from build123d import *

# Parameters (mm, degrees)
SKETCH1_R                = 95.25
BOSS_EXTRUDE1_DEPTH      = 482.6
SKETCH4_R                = 95.25
F_7_PERCENT_ULLAGE_DEPTH = 62.484


with BuildPart() as part:
    # Sketch1 → Boss-Extrude1 (new body)
    with BuildSketch(Plane(origin=(0, 0, 0), x_dir=(1, 0, 0), z_dir=(0, 1, 0))):
        Circle(SKETCH1_R)
    extrude(amount=BOSS_EXTRUDE1_DEPTH)

    # Sketch2 → Revolve1 (revolve)
    with BuildSketch(Plane(origin=(0, 0, 0), x_dir=(0, 0, -1), z_dir=(1, 0, 0))):
        with BuildLine():
            Line((0, 544.576), (0, 482.6))
            Line((0, 482.6), (95.25, 482.6))
            add(Edge.make_bspline(
                [(95.25, 482.6), (95.25, 544.576), (0, 544.576)],
                knots=[0, 0, 0, 1.570796327, 1.570796327, 1.570796327], degree=2, weights=[1, 0.707106781, 1]))
        make_face()
    revolve(axis=Axis((0, 544.576, 0), (0, -1, 0)))

    # Sketch3 → Revolve2 (revolve)
    with BuildSketch(Plane(origin=(0, 0, 0), x_dir=(0, 0, -1), z_dir=(1, 0, 0))):
        with BuildLine():
            Line((0, -59.69), (0, 0))
            Line((0, 0), (95.25, 0))
            add(Edge.make_bspline(
                [(0, -59.69), (95.25, -59.69), (95.25, 0)],
                knots=[4.71238898, 4.71238898, 4.71238898, 6.283185307, 6.283185307, 6.283185307], degree=2, weights=[1, 0.707106781, 1]))
        make_face()
    revolve(axis=Axis((0, -59.69, 0), (0, 1, 0)))

    # Sketch4 → 7 Percent Ullage (cut)
    with BuildSketch(Plane(origin=(0, 544.576, 0), x_dir=(1, 0, 0), z_dir=(0, 1, 0))):
        Circle(SKETCH4_R)
    extrude(amount=-F_7_PERCENT_ULLAGE_DEPTH, mode=Mode.SUBTRACT)


solid = part.part
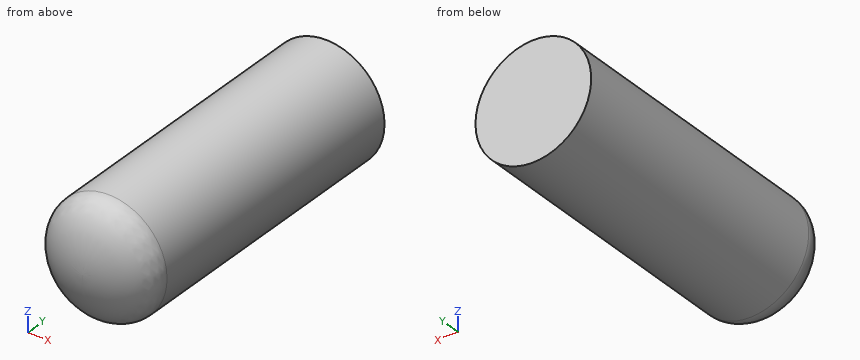
Work out the finished part from the listing and answer in its coordinate system (mm). Give positions to 0.01 mm unless a question says otherwise; leave off trailing zeros. Loops run counter-clockwise (first coordinate to the right, second up) from the corner with the lowest first, then second, coordinate; pieces in that order, holes last. Notation, with made-up numbers: (41, 55) - (99, 55) arc R12 cw to (99, 61) - close; hole circle Ø4 at (-35, -33.5). An arc over 180 degrees is marked (long way). Answer in a Markdown table with one row per item. Add a question column.
Q1. Consider line 1 along X through (y, z) = (93.5, 85); line 2 along X through (y, z) = (23.5, -68.5); line 3 along Z through (x, y) = (-79, 57.5). Determine where each line is inside the solid, lowest interval first.
Q2. Each of these flat-tipped pins is pushed along its axis until it touches: P1, Ø8, axis at x = 2.5, y = 119, coming from the +Z side; P2, Ø10, axis at y = 186.5, z = -30, coming from the +X side; P3, Ø8, axis at x = -53.5, y = 290, coming from the +Z side. Where does it stop, or does it pass through?
Q3. The part is cut by section A-A (y = 217). Determine the outline of the cut face in (x, z), and give its area (3 significant figures).
Solution:
| question | item | result |
|---|---|---|
| 1 | line 1 | x = -42.98 to 42.98 |
| 1 | line 2 | x = -66.18 to 66.18 |
| 1 | line 3 | z = -53.21 to 53.21 |
| 2 | P1 | stops at z = 95.25 |
| 2 | P2 | stops at x = 91.91 |
| 2 | P3 | stops at z = 81.38 |
| 3 | outline | circle Ø190.5 at (0, 0) |
| 3 | area | 28,500 mm² |
